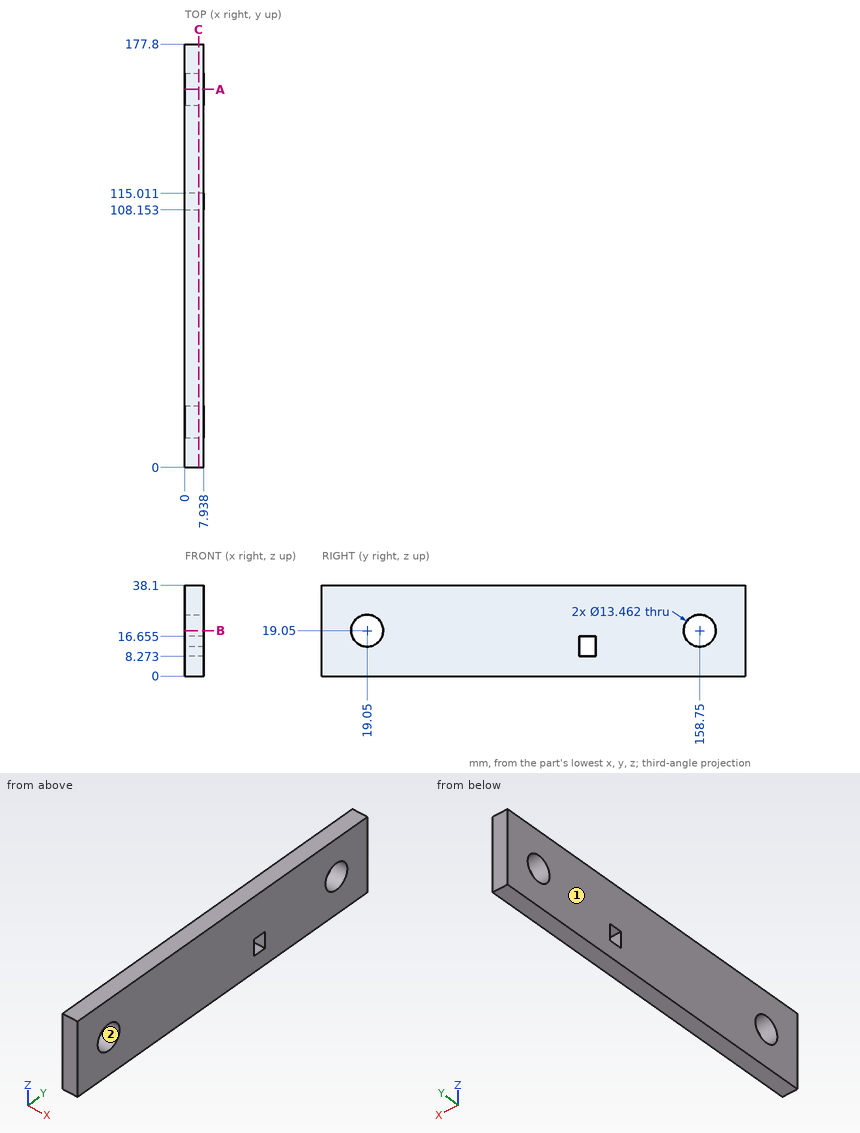
Input: dimensioned drawing with shaded views. Units: mm. Origin: part minimum x, y, z. Give positions to 0.01 mm unless a question says otherwise; leave off trailing zeros. Order: outer loops, then holes, each group sorted by start corner. A loop starts at its lowest first (then second) coordinate and runs counter-clockwise, first axis right, second up. Notation, with made-up numbers: (86.5, 9) -> (100.5, 9) arc R26 ccw to (100.5, 27) -> close; hole circle Ø2 at (44, -7.75). An arc over 180 degrees is marked (long way). Use one line per item in the form item = value.
1) Section C-C, the plane x = 5.75. Count the separate pieces of the cut face and the enclosed holes in it, and give its area (3 significant figures).
Response values:
separate_pieces = 1
enclosed_holes = 3
area = 6,430 mm^2
2) Section A-A, the plane y = 158.75. Return loops of the section in (x, z).
Response values:
outline = (0, 0) -> (7.94, 0) -> (7.94, 12.32) -> (0, 12.32) -> close; (0, 25.78) -> (7.94, 25.78) -> (7.94, 38.1) -> (0, 38.1) -> close
3) Line query: probe 1 along Y at (x, z) = (5.25, 19.05); probe 2 along Y at (x, z) = (2.25, 12); probe 3 along Z at (x, y) = (5.5, 158.75). Output: solid intervals per line, ascending.
Response values:
probe_1 = 0 to 12.32, 25.78 to 152.02, 165.48 to 177.8
probe_2 = 0 to 108.15, 115.01 to 177.8
probe_3 = 0 to 12.32, 25.78 to 38.1
4) First-contact query: pin 1 Ø4 at (y, z) = (34, 12) entering from -X. Flat tip, straight axial feed; report the tip coordinate or a pass-through.
Response values:
pin_1 = 0
5) Mould query, pull axis Z, two halves, no side actions, for the marked faces 1 and 2. Classes: pulls with the +Z half, pulls with the -Z half, needs draft (parallel to the pull), parting line crosses it, or undercut.
Response values:
face_1 = needs draft
face_2 = undercut
6) Section B-B, the plane z = 19.05. Return loops of the section in (x, y), and give its area (3 significant figures).
Response values:
outline = (0, 0) -> (7.94, 0) -> (7.94, 12.32) -> (0, 12.32) -> close; (0, 25.78) -> (7.94, 25.78) -> (7.94, 152.02) -> (0, 152.02) -> close; (0, 165.48) -> (7.94, 165.48) -> (7.94, 177.8) -> (0, 177.8) -> close
area = 1,200 mm^2
